```python
from build123d import *

# Parameters (mm, degrees)
F0_R     = 9.8568007518
F1_DEPTH = 25.4
F2_DEPTH = 145.2685


with BuildPart() as f1:
    # F0 (on Front) → F1 (new body)
    with BuildSketch(Plane.XZ):
        with BuildLine():
            ThreePointArc((18.574012772, -21.714895223), (25.954604986, -11.9536230918), (28.575, 0))
            ThreePointArc((28.575, 0), (20.2055762724, 20.2055762724), (0, 28.575))
            ThreePointArc((0, 28.575), (-28.575, 0), (0, -28.575))
            Line((0, -28.575), (18.574012772, -21.714895223))
        make_face()
        with BuildLine():
            ThreePointArc((-3.887280916, 9.0579008684), (0, 9.8568007518), (3.887280916, 9.0579008684))
            Line((3.887280916, 9.0579008684), (19.05, 9.0579008684))
            Line((19.05, 9.0579008684), (19.05, -9.0579008684))
            Line((19.05, -9.0579008684), (3.887280916, -9.0579008684))
            ThreePointArc((3.887280916, -9.0579008684), (0, -9.8568007518), (-3.887280916, -9.0579008684))
            Line((-3.887280916, -9.0579008684), (-19.05, -9.0579008684))
            Line((-19.05, -9.0579008684), (-19.05, 9.0579008684))
            Line((-19.05, 9.0579008684), (-3.887280916, 9.0579008684))
        make_face(mode=Mode.SUBTRACT)
        with BuildLine():
            ThreePointArc((0, 28.575), (20.2055762724, 20.2055762724), (28.575, 0))
            ThreePointArc((28.575, 0), (25.954604986, -11.9536230918), (18.574012772, -21.714895223))
            Line((18.574012772, -21.714895223), (55.185590913, -8.1928165434))
            ThreePointArc((55.185590913, -8.1928165434), (35.3722696716, 6.7149096533), (47.0745963207, 28.575))
            Line((47.0745963207, 28.575), (0, 28.575))
        make_face()
        with BuildLine():
            ThreePointArc((0, -28.575), (9.9001892407, -26.8051651366), (18.574012772, -21.714895223))
            Line((18.574012772, -21.714895223), (0, -28.575))
        make_face()
        with BuildLine():
            ThreePointArc((73.025, 10.81867918), (64.7325510668, 26.5405618613), (47.0745963207, 28.575))
            ThreePointArc((47.0745963207, 28.575), (35.3722696716, 6.7149096533), (55.185590913, -8.1928165434))
            ThreePointArc((55.185590913, -8.1928165434), (67.8668007633, -2.2166716612), (73.025, 10.81867918))
        make_face()
        with Locations((53.975, 10.81867918)):
            Circle(F0_R, mode=Mode.SUBTRACT)
        with BuildLine():
            Line((-3.887280916, 9.0579008684), (3.887280916, 9.0579008684))
            ThreePointArc((3.887280916, 9.0579008684), (0, 9.8568007518), (-3.887280916, 9.0579008684))
        make_face()
        with BuildLine():
            ThreePointArc((-3.887280916, -9.0579008684), (0, -9.8568007518), (3.887280916, -9.0579008684))
            Line((3.887280916, -9.0579008684), (-3.887280916, -9.0579008684))
        make_face()
        with BuildLine():
            ThreePointArc((-3.887280916, -9.0579008684), (-9.8568007518, 0), (-3.887280916, 9.0579008684))
            Line((-3.887280916, 9.0579008684), (-19.05, 9.0579008684))
            Line((-19.05, 9.0579008684), (-19.05, -9.0579008684))
            Line((-19.05, -9.0579008684), (-3.887280916, -9.0579008684))
        make_face()
    extrude(amount=F1_DEPTH)

    # F0 (on Front) → F2 (join)
    with BuildSketch(Plane.XZ):
        with BuildLine():
            ThreePointArc((18.574012772, -21.714895223), (25.954604986, -11.9536230918), (28.575, 0))
            ThreePointArc((28.575, 0), (20.2055762724, 20.2055762724), (0, 28.575))
            ThreePointArc((0, 28.575), (-28.575, 0), (0, -28.575))
            Line((0, -28.575), (18.574012772, -21.714895223))
        make_face()
        with BuildLine():
            ThreePointArc((-3.887280916, 9.0579008684), (0, 9.8568007518), (3.887280916, 9.0579008684))
            Line((3.887280916, 9.0579008684), (19.05, 9.0579008684))
            Line((19.05, 9.0579008684), (19.05, -9.0579008684))
            Line((19.05, -9.0579008684), (3.887280916, -9.0579008684))
            ThreePointArc((3.887280916, -9.0579008684), (0, -9.8568007518), (-3.887280916, -9.0579008684))
            Line((-3.887280916, -9.0579008684), (-19.05, -9.0579008684))
            Line((-19.05, -9.0579008684), (-19.05, 9.0579008684))
            Line((-19.05, 9.0579008684), (-3.887280916, 9.0579008684))
        make_face(mode=Mode.SUBTRACT)
        with BuildLine():
            ThreePointArc((-3.887280916, -9.0579008684), (-9.8568007518, 0), (-3.887280916, 9.0579008684))
            Line((-3.887280916, 9.0579008684), (-19.05, 9.0579008684))
            Line((-19.05, 9.0579008684), (-19.05, -9.0579008684))
            Line((-19.05, -9.0579008684), (-3.887280916, -9.0579008684))
        make_face()
    extrude(amount=F2_DEPTH)


solid = f1.part
```
The model under review builds one solid part; all positions refer to its coordinate system, in mm. A direction names the side the tool comes from. Give positions to 0.01 mm unless a question says otherwise; leave off trailing zeros. Write each loop counter-clockwise with the first axis right and the second up, starting at its lowest first coordinate (ties: lowest second). Pieces come first, ordered by that corner, then holes.
(1) Consider section B-B, the plane z = -1.5. Give the boundary of the cut face in (x, y).
(2) Tool access review of faces 1 (the cylindrical face through (-9.853, -71.617, -0.273)), 2 (the flat face through (24, -13, 28.575)), 3 (the flat face through (19.05, -72, 0)): name each direction out of +Z, -Z, +X, -X, +Y, -Y from which nothing blocks a thin tool from reaching the whole face with its end or side.
(3) Consider section A-A, the plane x = 11.5. Give the boundary of the cut face in (y, z) (1 decimal), and give its area (3 significant figures).
(4) Consider section C-C, the plane y = -48. Give the boundary of the cut face in (x, z) (3 decimals).
(5) To check wall thickness, follow L1, parallel to X at y = -84, z = 0 (3 decimals); L2, parallel to X at y = -16, z = 7.5; L3, parallel to X at y = -121, z = -5.5. State the ranges of each line that lie inside material, in increasing order.
(6) For P1, Ø2, axis at y = -62.5, z = 16.5, coming from the +X side; P2, Ø8, axis at x = 27, y = -21, coming from the -Z side; P3, Ø18.5, axis at x = 2.5, y = -65, coming from the +Z side (3 decimals), all flat-tipped, find the tip position at first contact; note any pin that passes through.
(7) The part is to be moulded in two halves that separate along X. For faces 4 (the flat face through (10, -72, 9.058)), 5 (the flat face through (10, -72, -9.058)), 6 (the flat face through (22, 0, 1)), 7 (the flat face through (9.16, -84.5, -25.19)), say which applies: released by +X, released by -X, zero draft, split by the parting line, or undercut.
(8) Consider section D-D, the plane x = 62. Give the boundary of the cut face in (y, z).
Returned:
1. outline: (-28.54, -145.27) - (-9.74, -145.27) - (-9.74, 0) - (-28.54, 0) - close; (19.05, -145.27) - (28.54, -145.27) - (28.54, -25.4) - (68.51, -25.4) - (68.51, 0) - (19.05, 0) - close
2. face 1: -Y
2. face 2: +Z, -X, +Y, -Y
2. face 3: +Y, -Y
3. outline: (-145.3, -24.3) - (-25.4, -24.3) - (-25.4, -26.2) - (0, -26.2) - (0, -9.1) - (-145.3, -9.1) - close; (-145.3, 9.1) - (0, 9.1) - (0, 28.6) - (-25.4, 28.6) - (-25.4, 26.2) - (-145.3, 26.2) - close
3. area: 4,810 mm2
4. outline: (0, -28.575) - (18.574, -21.715) arc R28.575 ccw (long way) to start; hole (3.887, -9.058) - (19.05, -9.058) - (19.05, 9.058) - (3.887, 9.058) arc R9.857 ccw (long way) to start
5. L1: x = -28.575 to -9.857, 19.05 to 28.575
5. L2: x = -27.57 to -6.4, 19.05 to 44.69, 63.26 to 72.73
5. L3: x = -28.04 to -8.18, 19.05 to 28.04
6. P1: stops at x = 24.01
6. P2: stops at z = -20.08
6. P3: stops at z = 28.575
7. face 4: undercut
7. face 5: undercut
7. face 6: zero draft
7. face 7: released by +X
8. outline: (-25.4, -6.46) - (0, -6.46) - (0, 5.1) - (-25.4, 5.1) - close; (-25.4, 16.54) - (0, 16.54) - (0, 28.1) - (-25.4, 28.1) - close
